from build123d import *

# Parameters (mm, degrees)
SKETCH1_R      = 1.6
EXTRUDE1_DEPTH = 10
EXTRUDE2_DEPTH = 10
SKETCH3_R      = 3.75
EXTRUDE3_DEPTH = 10
SKETCH4_W      = 29.5
SKETCH4_H      = 13
EXTRUDE4_DEPTH = 9.2
SKETCH5_W      = 29.5
SKETCH5_H      = 8.4
EXTRUDE5_DEPTH = 4.3
SKETCH6_W      = 7.5
SKETCH6_H      = 7.2
SKETCH6_W_2    = 16.3
EXTRUDE6_DEPTH = 2
SKETCH7_W      = 10.1
SKETCH7_H      = 8
EXTRUDE7_DEPTH = 12.5


with BuildPart() as part:
    # Sketch1 → Extrude1 (new body)
    with BuildSketch(Plane(origin=(0, 0, 0), x_dir=(1, 0, 0), z_dir=(0, 1, 0))):
        with BuildLine():
            Line((-18.5, -3.75), (18.5, -3.75))
            ThreePointArc((18.5, -3.75), (22.25, 0), (18.5, 3.75))
            Line((18.5, 3.75), (-18.5, 3.75))
            ThreePointArc((-18.5, 3.75), (-22.25, 0), (-18.5, -3.75))
        make_face()
        with Locations(Location((18.5, 0, 0), (0, 0, 270))):
            Circle(SKETCH1_R, mode=Mode.SUBTRACT)
        with Locations(Location((-18.5, 0, 0), (0, 0, 270))):
            Circle(SKETCH1_R, mode=Mode.SUBTRACT)
    extrude(amount=EXTRUDE1_DEPTH)

    # Sketch2 → Extrude2 (cut)
    with BuildSketch(Plane.XY.offset(3.75)):
        Polygon((-22.25, 2), (-18.5, 2), (-10.5, 10), (10.5, 10), (18.5, 2), (22.25, 2), (22.25, 12), (-22.25, 12), align=None)
    extrude(amount=-EXTRUDE2_DEPTH, mode=Mode.SUBTRACT)

    # Sketch3 → Extrude3 (cut)
    with BuildSketch(Plane(origin=(0, 2, 0), x_dir=(1, 0, 0), z_dir=(0, 1, 0))):
        with Locations((-18.5, 0)):
            Circle(SKETCH3_R)
        with Locations((18.5, 0)):
            Circle(SKETCH3_R)
    extrude(amount=EXTRUDE3_DEPTH, mode=Mode.SUBTRACT)

    # Sketch4 → Extrude4 (add)
    with BuildSketch(Plane.XZ):
        Rectangle(SKETCH4_W, SKETCH4_H)
    extrude(amount=-EXTRUDE4_DEPTH)

    # Sketch5 → Extrude5 (add)
    with BuildSketch(Plane(origin=(0, 9.2, 0), x_dir=(1, 0, 0), z_dir=(0, 1, 0))):
        Rectangle(SKETCH5_W, SKETCH5_H)
    extrude(amount=EXTRUDE5_DEPTH)

    # Sketch6 → Extrude6 (add)
    with BuildSketch(Plane(origin=(0, 13.5, 0), x_dir=(1, 0, 0), z_dir=(0, 1, 0))):
        with Locations((-10.25, 0)):
            Rectangle(SKETCH6_W, SKETCH6_H)
        with Locations((5.85, 0)):
            Rectangle(SKETCH6_W_2, SKETCH6_H)
    extrude(amount=EXTRUDE6_DEPTH)

    # Sketch7 → Extrude7 (add)
    with BuildSketch(Plane.XY):
        with Locations((0, 7.3)):
            Rectangle(SKETCH7_W, SKETCH7_H)
    extrude(amount=EXTRUDE7_DEPTH)


solid = part.part
Geometry check sheet. Reference: the model listing, model coordinates, mm. A direction names the side the tool comes from. Round coordinates to 2 decimals unless told otherwise and drop trailing zeros. Loops run counter-clockwise (first coordinate to the right, second up) from the corner with the lowest first, then second, coordinate; pieces in that order, holes last.
Item 1: Mould release check, pull along Z, two halves, no side actions. Record for faces 5 (the cylindrical face through (-16.914, 0.986, -0.208)), 6 (the flat face through (-19, 2, -2)), 7 (the flat face through (-16, 2, -3.75)), 8 (the flat face through (-14.75, 7, 0)): pulls with the +Z half, pulls with the -Z half, needs draft (parallel to the pull), parting line crosses it, or undercut.
Item 2: Gauge pin test, flat ends, axial feed: pin 1 (0.7 mm diameter, centred on x = -8, z = 5, fed in from +Y); pin 2 (1.9 mm diameter, centred on x = 16.5, y = 4, fed in from +Z); pin 3 (2 mm diameter, centred on x = 4.5, y = 12, fed in from -Z); pin 4 (3 mm diameter, centred on x = 18.5, z = 0, fed in from -Y). Record the tip position at first contact, or that the pin passes through.
Item 3: Cross-section at C-C on y = 4.5. Record the boundary of the cut face in (x, z), then the cut area to 3 significant figures.
Item 4: Access from +Z, -Z, +X, -X, +Y, -Y to the whole of each face (thin tool, end or side, straight path). Record for faces 1 (the flat face through (-14, 14, 0)), 2 (the flat face through (-10, 14, 3.6)), 3 (the flat face through (-2.3, 14, 0)), 4 (the cylindrical face through (14.75, 3.43, -0.08)).
Item 5: Cross-section at A-A on y = 9.75. Record the boundary of the cut face in (x, z).
Item 6: Thickness scan on line 1 (X direction, y = 0.95, z = 0); line 2 (Y direction, x = 1, z = -4); line 3 (X direction, y = 7.5, z = 0.5). Record the ranges inside material, lowest first.
Item 7: Cross-section at B-B on z = 7.5. Record the boundary of the cut face in (x, y).
Item 8: Cross-section at D-D on z = -4.75. Record the boundary of the cut face in (x, y), then the cut area to 3 significant figures.
Answer sheet:
1. face 5: undercut
1. face 6: undercut
1. face 7: pulls with the -Z half
1. face 8: needs draft
2. pin 1: stops at y = 9.2
2. pin 2: stops at z = 3.75
2. pin 3: stops at z = -4.2
2. pin 4: passes through
3. outline: (-16, -3.75) - (-14.75, -3.75) - (-14.75, -6.5) - (14.75, -6.5) - (14.75, -3.75) - (16, -3.75) - (16, -2.8) arc R3.75 cw to (16, 2.8) - (16, 3.75) - (14.75, 3.75) - (14.75, 6.5) - (5.05, 6.5) - (5.05, 12.5) - (-5.05, 12.5) - (-5.05, 6.5) - (-14.75, 6.5) - (-14.75, 3.75) - (-16, 3.75) - (-16, 2.8) arc R3.75 cw to (-16, -2.8) - close
3. area: 453 mm2
4. face 1: +Z, -Z, -X, +Y
4. face 2: +Z, +X, -X, +Y
4. face 3: +Z, -Z, +Y
4. face 4: +X, +Y
5. outline: (-14.75, -4.2) - (14.75, -4.2) - (14.75, 4.2) - (5.05, 4.2) - (5.05, 12.5) - (-5.05, 12.5) - (-5.05, 4.2) - (-14.75, 4.2) - close
6. line 1: x = -22.25 to -20.1, -16.9 to 16.9, 20.1 to 22.25
6. line 2: y = 0 to 13.5
6. line 3: x = -14.75 to 14.75
7. outline: (-5.05, 3.3) - (5.05, 3.3) - (5.05, 11.3) - (-5.05, 11.3) - close
8. outline: (-14.75, 0) - (14.75, 0) - (14.75, 9.2) - (-14.75, 9.2) - close
8. area: 271 mm2
